Source: three-view drawing plus pictorial views. Frame: mm from the lowest corner of the part. Give positions to 0.01 mm unless a question says otherwise; leave off trailing zeros. Loops run counter-clockwise (first coordinate to the right, second up) from the corner with the lowest first, then second, coordinate; pieces in that order, holes last. Notation, with made-up numbers: M 36.25,-36 L 55.25,-36 A10 cw 55.25,-32 Z; hole C -4.5,-24.5 d7. An arc over 180 degrees is marked long. Write item = value, one per line.
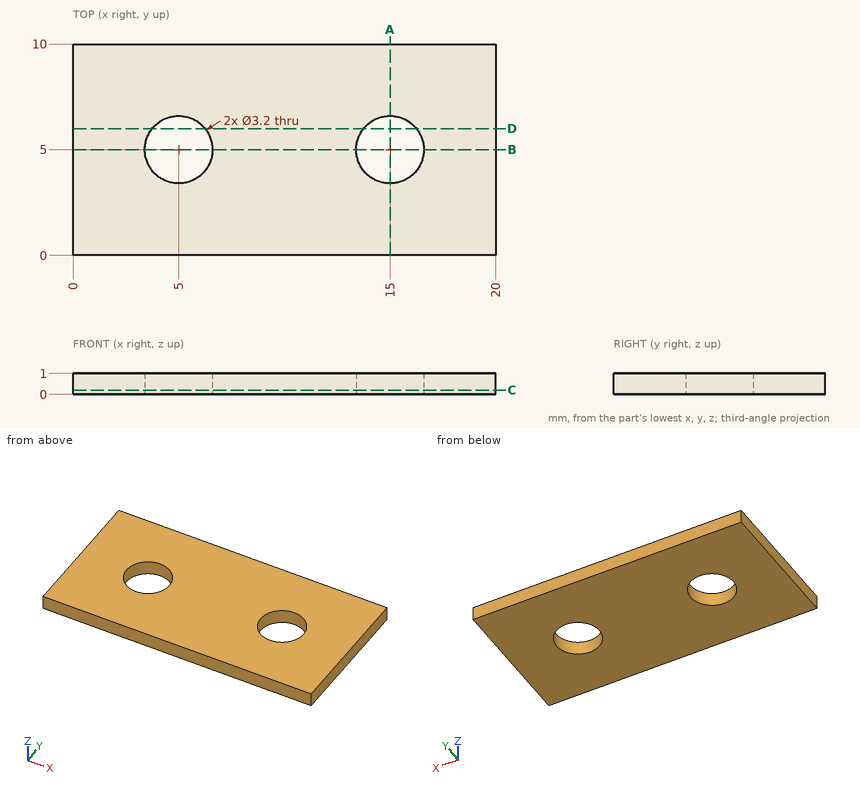
1. First-contact query: pin 1 Ø3 at (x, y) = (5, 5) entering from +Z. Flat tip, straight axial feed; report the tip coordinate or a pass-through.
Derived:
pin_1 = through
2. Cut plane A-A, the plane x = 15. Return the cut outline in (y, z).
Derived:
outline = M 0,0 L 3.4,0 L 3.4,1 L 0,1 Z; M 6.6,0 L 10,0 L 10,1 L 6.6,1 Z
3. Cut plane B-B, the plane y = 5. Return the cut outline in (x, z), then the cut area to 3 significant figures.
Derived:
outline = M 0,0 L 3.4,0 L 3.4,1 L 0,1 Z; M 6.6,0 L 13.4,0 L 13.4,1 L 6.6,1 Z; M 16.6,0 L 20,0 L 20,1 L 16.6,1 Z
area = 13.6 mm²
4. Cut plane D-D, the plane y = 6. Return the cut outline in (x, z).
Derived:
outline = M 0,0 L 3.75,0 L 3.75,1 L 0,1 Z; M 6.25,0 L 13.75,0 L 13.75,1 L 6.25,1 Z; M 16.25,0 L 20,0 L 20,1 L 16.25,1 Z
5. Cut plane C-C, the plane z = 0.2. Return the cut outline in (x, y).
Derived:
outline = M 0,0 L 20,0 L 20,10 L 0,10 Z; hole C 5,5 d3.2; hole C 15,5 d3.2
6. Material intervals for probe 1 along X at (y, z) = (5, 0.7); probe 2 along Y at (x, z) = (5, 0.85); probe 3 along X at (y, z) = (5.5, 0.35), sorted ascending. Write a range as from..to.
Derived:
probe_1 = 0..3.4, 6.6..13.4, 16.6..20
probe_2 = 0..3.4, 6.6..10
probe_3 = 0..3.48, 6.52..13.48, 16.52..20
